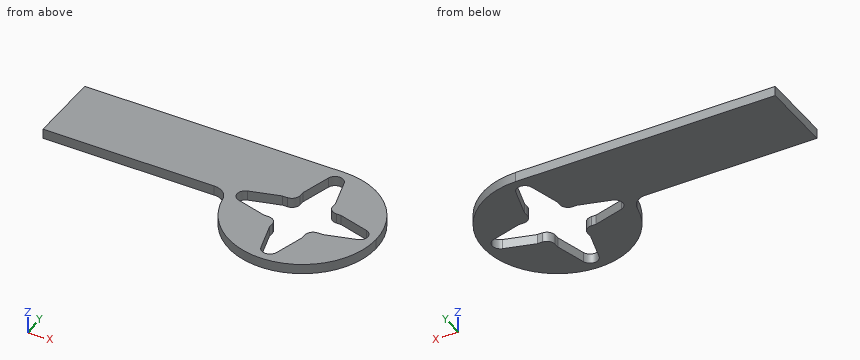
```python
from build123d import *

# Parameters (mm, degrees)
SKETCH1_R           = 2.5
SKETCH1_W           = 57
SKETCH1_H           = 22.5
BOSS_EXTRUDE1_DEPTH = 3


with BuildPart() as part:
    # Sketch1 → Boss-Extrude1 (new body)
    # profile 1 of 8: a face of its own
    with BuildSketch(Plane.XY):
        with BuildLine():
            ThreePointArc((22.5, 0), (15.909902577, 15.909902577), (0, 22.5))
            Line((0, 22.5), (-22.5, 0))
            Line((-22.5, 0), (-22.124973736, -4.090909091))
            ThreePointArc((-22.124973736, -4.090909091), (2.054031517, -22.406047276), (22.5, 0))
        make_face()
        with BuildLine():
            ThreePointArc((-7.5, 5), (-9.267766953, 9.267766953), (-5, 7.5))
            Line((-5, 7.5), (-5, 9))
            Line((-5, 9), (-2.405779746, 18.179870439))
            ThreePointArc((-2.405779746, 18.179870439), (0, 20), (2.405779746, 18.179870439))
            Line((2.405779746, 18.179870439), (5, 9))
            Line((5, 9), (5, 7.5))
            ThreePointArc((5, 7.5), (7.5, 10), (10, 7.5))
            ThreePointArc((10, 7.5), (9.267766953, 5.732233047), (7.5, 5))
            Line((7.5, 5), (9, 5))
            Line((9, 5), (18.179870439, 2.405779746))
            ThreePointArc((18.179870439, 2.405779746), (19.493699588, 1.508363998), (20, 0))
            ThreePointArc((20, 0), (19.493699588, -1.508363998), (18.179870439, -2.405779746))
            Line((18.179870439, -2.405779746), (9, -5))
            Line((9, -5), (7.5, -5))
            ThreePointArc((7.5, -5), (9.267766953, -5.732233047), (10, -7.5))
            ThreePointArc((10, -7.5), (7.5, -10), (5, -7.5))
            Line((5, -7.5), (5, -9))
            Line((5, -9), (2.405779746, -18.179870439))
            ThreePointArc((2.405779746, -18.179870439), (0, -20), (-2.405779746, -18.179870439))
            Line((-2.405779746, -18.179870439), (-5, -9))
            Line((-5, -9), (-5, -7.5))
            ThreePointArc((-5, -7.5), (-9.267766953, -9.267766953), (-7.5, -5))
            Line((-7.5, -5), (-9, -5))
            Line((-9, -5), (-18.179870439, -2.405779746))
            ThreePointArc((-18.179870439, -2.405779746), (-20, 0), (-18.179870439, 2.405779746))
            Line((-18.179870439, 2.405779746), (-9, 5))
            Line((-9, 5), (-7.5, 5))
        make_face(mode=Mode.SUBTRACT)
    # profile 2 of 8: a face of its own
    with BuildSketch(Plane.XY):
        with Locations((-7.5, 7.5)):
            Circle(SKETCH1_R)
    # profile 3 of 8: a face of its own
    with BuildSketch(Plane.XY):
        with Locations((7.5, 7.5)):
            Circle(SKETCH1_R)
    # profile 4 of 8: a face of its own
    with BuildSketch(Plane.XY):
        with Locations((7.5, -7.5)):
            Circle(SKETCH1_R)
    # profile 5 of 8: a face of its own
    with BuildSketch(Plane.XY):
        with Locations((-7.5, -7.5)):
            Circle(SKETCH1_R)
    # profile 6 of 8: a face of its own
    with BuildSketch(Plane.XY):
        Polygon((-22.5, 22.5), (0, 22.5), (-22.5, 0), align=None)
    # profile 7 of 8: a face of its own
    with BuildSketch(Plane.XY):
        with Locations((-51, 11.25)):
            Rectangle(SKETCH1_W, SKETCH1_H)
    # profile 8 of 8: a face of its own
    with BuildSketch(Plane.XY):
        with BuildLine():
            Line((-22.5, 0), (-22.124973736, -4.090909091))
            ThreePointArc((-22.124973736, -4.090909091), (-23.843623821, -1.156469426), (-27.041634566, 0))
            Line((-27.041634566, 0), (-22.5, 0))
        make_face()
    extrude(amount=BOSS_EXTRUDE1_DEPTH)


solid = part.part
```
CAD build for the part. Positions are in the model's coordinates, mm. Round coordinates to 2 decimals unless told otherwise and drop trailing zeros. Order: outer loops, then holes, each group sorted by start corner. A loop starts at its lowest first (then second) coordinate and runs counter-clockwise, first axis right, second up. Notation, with made-up numbers: (50.25, 25) - (81.25, 25) arc R16 cw to (81.25, 36) - close; hole circle Ø10 at (-3.5, 11). An arc over 180 degrees is marked (long way). Answer in a Markdown table with one row per item. Add a question column.
(1) Drop flat-ended pins along their axis: pin 1 Ø1.6 at (x, z) = (8, 1) entering from +Y; pin 2 Ø1.6 at (y, z) = (-8.5, 2) entering from +X; pin 3 Ø1.2 at (x, z) = (-8.5, 2) entering from -Y. Give the stop position or say it passes through.
(2) Band-saw the part on B-B on x = 11. List the corners of the cut face in (y, z).
(3) Band-saw the part on D-D on x = -52.5. List the corners of the cut face in (y, z).
(4) Band-saw the part on C-C on y = 1.5. List the corners of the cut face in (x, z).
(5) Probe L1, parallel to Y at x = -74, z = 1.2; L2, parallel to X at y = 14, z = 1.55; L3, parallel to X at y = -7, z = 1.55. List the from-to ranges inside material, lowest first. Write a range as [from, to].
Data:
| question | item | result |
|---|---|---|
| 1 | pin 1 | stops at y = 21.32 |
| 1 | pin 2 | stops at x = 21.14 |
| 1 | pin 3 | stops at y = -21.07 |
| 2 | outline | (-19.63, 0) - (-4.43, 0) - (-4.43, 3) - (-19.63, 3) - close; (4.43, 0) - (19.63, 0) - (19.63, 3) - (4.43, 3) - close |
| 3 | outline | (0, 0) - (22.5, 0) - (22.5, 3) - (0, 3) - close |
| 4 | outline | (-79.5, 0) - (-19.5, 0) - (-19.5, 3) - (-79.5, 3) - close; (19.5, 0) - (22.45, 0) - (22.45, 3) - (19.5, 3) - close |
| 5 | L1 | y = [0, 22.5] |
| 5 | L2 | x = [-79.5, -3.59], [3.59, 17.61] |
| 5 | L3 | x = [-21.38, -5.05], [5.05, 21.38] |
